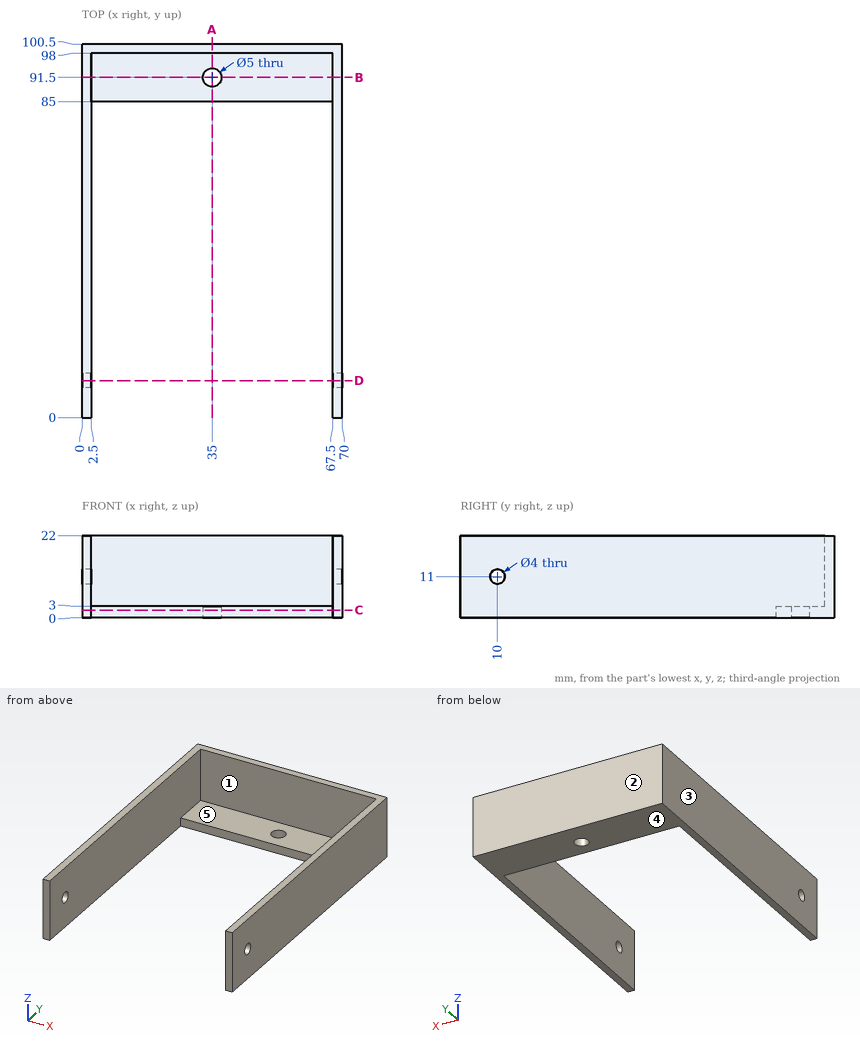
For this review, use the dimensioned drawing (mm, ordinates from the lowest corner) and the shaded views. A direction names the side the tool comes from. Round coordinates to 2 decimals unless told otherwise and drop trailing zeros. Order: outer loops, then holes, each group sorted by start corner. A loop starts at its lowest first (then second) coordinate and runs counter-clockwise, first axis right, second up. Notation, with made-up numbers: (30, -10.75) -> (51, -10.75) arc R24 cw to (51, 12.25) -> close; hole circle Ø7 at (81, 78.5). An arc over 180 degrees is marked (long way). Put each result on its own line as item: value.
Q1. Add section D-D on y = 10. Write out the cut boundary in (x, z), plus the area to 3 significant figures.
Check result:
outline: (0, 0) -> (2.5, 0) -> (2.5, 9) -> (0, 9) -> close; (0, 13) -> (2.5, 13) -> (2.5, 22) -> (0, 22) -> close; (67.5, 0) -> (70, 0) -> (70, 9) -> (67.5, 9) -> close; (67.5, 13) -> (70, 13) -> (70, 22) -> (67.5, 22) -> close
area: 90.0 mm2
Q2. Add section B-B on y = 91.5. Write out the cut boundary in (x, z).
Check result:
outline: (0, 0) -> (32.5, 0) -> (32.5, 3) -> (2.5, 3) -> (2.5, 22) -> (0, 22) -> close; (37.5, 0) -> (70, 0) -> (70, 22) -> (67.5, 22) -> (67.5, 3) -> (37.5, 3) -> close
Q3. Mouldability with a two-part tool opening along X and no side actions: class the marked faces 1, 2 and 3 as pulls with the +X half, pulls with the -X half, needs draft (parallel to the pull), parting line crosses it, or undercut.
Check result:
face 1: undercut
face 2: needs draft
face 3: pulls with the -X half
Q4. Insertion check: pin 1 Ø6 at (x, z) = (60, 9.5) entering from -Y; pin 2 Ø5 at (y, z) = (10, 11) entering from -X; pin 3 Ø8 at (x, y) = (35, 91.5) entering from +Z; pin 4 Ø2.5 at (x, z) = (37.5, 1.5) entering from -Y. Each pin has a flat end and moves straight along its axis. Give the tip position at first contact, or say it passes through.
Check result:
pin 1: y = 98
pin 2: x = 0
pin 3: z = 3
pin 4: y = 85
Q5. Machinability: for the marked faces 4 and 5, which of the approach directions +Z, -Z, +X, -X, +Y, -Y give a long, thin tool a straight path to every point of the face, cutting with its end or side? Answer none if there is none.
Check result:
face 4: -Z, +X, -X, +Y, -Y
face 5: +Z, -Y
Q6. Add section C-C on z = 2. Write out the cut boundary in (x, y).
Check result:
outline: (0, 0) -> (2.5, 0) -> (2.5, 85) -> (67.5, 85) -> (67.5, 0) -> (70, 0) -> (70, 100.5) -> (0, 100.5) -> close; hole circle Ø5 at (35, 91.5)
Q7. Add section A-A on x = 35. Write out the cut boundary in (y, z), plus the area to 3 significant figures.
Check result:
outline: (85, 0) -> (89, 0) -> (89, 3) -> (85, 3) -> close; (94, 0) -> (100.5, 0) -> (100.5, 22) -> (98, 22) -> (98, 3) -> (94, 3) -> close
area: 79.0 mm2
Q8. For probe 1 along X at (y, z) = (95.5, 17.75); probe 2 along X at (y, z) = (91.5, 0.8); probe 3 along Y at (x, z) = (46, 3.75), list the stretches that pass through material, from the lowest coordinate up. Write a range as [from, to].
Check result:
probe 1: [0, 2.5], [67.5, 70]
probe 2: [0, 32.5], [37.5, 70]
probe 3: [98, 100.5]
